```python
from build123d import *

# Parameters (mm, degrees)
ESQUISSE1_W             = 130.51
ESQUISSE1_H             = 72.96
BOSS_EXTRU_4_DEPTH      = 4
ESQUISSE5_W             = 128.51
ESQUISSE5_H             = 70.96
ENL_V_MAT_EXTRU_1_DEPTH = 1.36
ESQUISSE6_W             = 60.96
ESQUISSE6_H             = 1.36
ENL_V_MAT_EXTRU_2_DEPTH = 149.70104808
ESQUISSE12_W            = 5.045005
ESQUISSE12_H            = 5
BOSS_EXTRU_10_DEPTH     = 4
ESQUISSE14_W            = 2
ESQUISSE14_H            = 5
BOSS_EXTRU_11_DEPTH     = 8
ESQUISSE15_W            = 2
ESQUISSE15_H            = 6
BOSS_EXTRU_12_DEPTH     = 8
ESQUISSE16_W            = 2
ESQUISSE16_H            = 6
BOSS_EXTRU_13_DEPTH     = 8
ESQUISSE17_W            = 5.045005
ESQUISSE17_H            = 5
BOSS_EXTRU_14_DEPTH     = 4
ESQUISSE19_W            = 2
ESQUISSE19_H            = 5
BOSS_EXTRU_15_DEPTH     = 8


with BuildPart() as part:
    # Esquisse1 → Boss.-Extru.4 (new body)
    with BuildSketch(Plane(origin=(0, 0, 0), x_dir=(1, 0, 0), z_dir=(0, 1, 0))):
        with Locations((65.255, 36.48)):
            Rectangle(ESQUISSE1_W, ESQUISSE1_H)
    extrude(amount=BOSS_EXTRU_4_DEPTH)

    # Esquisse5 → Enlèv. mat.-Extru.1 (cut)
    with BuildSketch(Plane(origin=(0, 4, 0), x_dir=(1, 0, 0), z_dir=(0, 1, 0))):
        with Locations((65.255, 36.48)):
            Rectangle(ESQUISSE5_W, ESQUISSE5_H)
    extrude(amount=-ENL_V_MAT_EXTRU_1_DEPTH, mode=Mode.SUBTRACT)

    # Esquisse6 → Enlèv. mat.-Extru.2 (cut, through all)
    with BuildSketch(Plane.ZY.offset(-129.51)):
        with Locations((-36.48, 3.32)):
            Rectangle(ESQUISSE6_W, ESQUISSE6_H)
    extrude(amount=-ENL_V_MAT_EXTRU_2_DEPTH, mode=Mode.SUBTRACT)

    # Esquisse12 → Boss.-Extru.10 (add)
    with BuildSketch(Plane.XZ):
        with Locations((133.0325025, -70.46)):
            Rectangle(ESQUISSE12_W, ESQUISSE12_H)
        with Locations((133.0325025, -2.5)):
            Rectangle(ESQUISSE12_W, ESQUISSE12_H)
    extrude(amount=-BOSS_EXTRU_10_DEPTH)

    # Esquisse14 → Boss.-Extru.11 (add)
    with BuildSketch(Plane(origin=(0, 4, 0), x_dir=(1, 0, 0), z_dir=(0, 1, 0))):
        with Locations((134.555005, 70.46)):
            Rectangle(ESQUISSE14_W, ESQUISSE14_H)
        with Locations((134.555005, 2.5)):
            Rectangle(ESQUISSE14_W, ESQUISSE14_H)
    extrude(amount=BOSS_EXTRU_11_DEPTH)

    # Esquisse15 → Boss.-Extru.12 (add)
    with BuildSketch(Plane(origin=(0, 0, -5), x_dir=(-1, 0, 0), z_dir=(0, 0, -1))):
        with Locations((-134.555005, 9)):
            Rectangle(ESQUISSE15_W, ESQUISSE15_H)
    extrude(amount=BOSS_EXTRU_12_DEPTH)

    # Esquisse16 → Boss.-Extru.13 (add)
    with BuildSketch(Plane.XY.offset(-67.96)):
        with Locations((134.555005, 9)):
            Rectangle(ESQUISSE16_W, ESQUISSE16_H)
    extrude(amount=BOSS_EXTRU_13_DEPTH)

    # Esquisse17 → Boss.-Extru.14 (add)
    with BuildSketch(Plane.XZ):
        with Locations((-2.5225025, -52.46)):
            Rectangle(ESQUISSE17_W, ESQUISSE17_H)
        with Locations((-2.5225025, -20.5)):
            Rectangle(ESQUISSE17_W, ESQUISSE17_H)
    extrude(amount=-BOSS_EXTRU_14_DEPTH)

    # Esquisse19 → Boss.-Extru.15 (add)
    with BuildSketch(Plane(origin=(0, 4, 0), x_dir=(1, 0, 0), z_dir=(0, 1, 0))):
        with Locations((-4.045005, 52.46)):
            Rectangle(ESQUISSE19_W, ESQUISSE19_H)
        with Locations((-4.045005, 20.5)):
            Rectangle(ESQUISSE19_W, ESQUISSE19_H)
    extrude(amount=BOSS_EXTRU_15_DEPTH)


solid = part.part
```
The listing builds one solid part. Answer for the finished solid, in the listing's coordinates (mm). A direction names the side the tool comes from. Coordinates: 2 decimals unless noted, no trailing zeros. Write each loop counter-clockwise with the first axis right and the second up, starting at its lowest first coordinate (ties: lowest second). Pieces come first, ordered by that corner, then holes. Notation, with made-up numbers: M 41,58.25 L 74,58.25 A37 cw 74,96.25 Z; hole C 35,80.25 d8. An arc over 180 degrees is marked long. Use a Markdown table: item, result. Add a question column.
1. Section C-C (x = 73) is taken. Give the vertices of the cut face in (y, z), plus the area to 3 significant figures.
2. Given P1, Ø5.5, axis at x = -1.5, y = 6.5, coming from the -Z side; P2, Ø1.6, axis at x = 135, z = -65.5, coming from the -Y side; P3, Ø2, axis at y = 2.5, z = -32, coming from the -X side; P4, Ø1.5, axis at x = 16, z = -33.5, coming from the -Y side, each flat-ended and moving along its own axis, determine where each tip first touches the part or whether it passes through.
3. Section D-D (z = -48) is taken. Give the vertices of the cut face in (x, y), plus the area to 3 significant figures.
4. Straight lines are drawn through the part: line 1 along Z through (x, y) = (59.5, 3.75); line 2 along X through (y, z) = (3.25, -68) (3 decimals); line 3 along Y through (x, z) = (14, -6.5). For each, find the intervals that lie inside material, in ascending order. Write a range as [from, to].
5. Which of the six approach directions +Z, -Z, +X, -X, +Y, -Y give full straight-line access (tool end or side, diameter ignored) to faces 1 (the flat face through (-4, 5, -23)), 2 (the flat face through (130.51, 1, -36)), 3 (the flat face through (0, 2, -64)), 4 (the flat face through (-3.045, 8, -52))?
6. Section B-B (z = -63.5) is taken. Give the vertices of the cut face in (x, y) (3 decimals).
7. Section A-A (y = 9) is taken. Give the vertices of the cut face in (x, z) (3 decimals).
8. For a pull along Z with two mould halves and no side action, classify faces 5 (the flat face through (0, 2, -9)), 6 (the flat face through (-4, 5, -54.96)), 7 (the flat face through (133, 2, -5)) as +Z half, -Z half, draft (parallel to the pull), parting line (faces both ways), or undercut.
Data:
| question | item | result |
|---|---|---|
| 1 | outline | M 0,-72.96 L 4,-72.96 L 4,-71.96 L 2.64,-71.96 L 2.64,-1 L 4,-1 L 4,0 L 0,0 Z |
| 1 | area | 195 mm2 |
| 2 | P1 | stops at z = -54.96 |
| 2 | P2 | stops at y = 6 |
| 2 | P3 | stops at x = 0 |
| 2 | P4 | stops at y = 0 |
| 3 | outline | M 0,0 L 130.51,0 L 130.51,2.64 L 1,2.64 L 1,4 L 0,4 Z |
| 3 | area | 346 mm2 |
| 4 | line 1 | z = [-72.96, -71.96], [-1, 0] |
| 4 | line 2 | x = [0, 1], [129.51, 135.555] |
| 4 | line 3 | y = [0, 2.64] |
| 5 | face 1 | -X, +Y, -Y |
| 5 | face 2 | +X, +Y, -Y |
| 5 | face 3 | -Z, -X, +Y, -Y |
| 5 | face 4 | +Z, -Z, +X, +Y |
| 6 | outline | M 0,0 L 130.51,0 L 130.51,2.64 L 1,2.64 L 1,4 L 0,4 Z; M 133.555,6 L 135.555,6 L 135.555,12 L 133.555,12 Z |
| 7 | outline | M -5.045,-54.96 L -3.045,-54.96 L -3.045,-49.96 L -5.045,-49.96 Z; M -5.045,-23 L -3.045,-23 L -3.045,-18 L -5.045,-18 Z; M 133.555,-72.96 L 135.555,-72.96 L 135.555,-59.96 L 133.555,-59.96 Z; M 133.555,-13 L 135.555,-13 L 135.555,0 L 133.555,0 Z |
| 8 | face 5 | draft |
| 8 | face 6 | -Z half |
| 8 | face 7 | undercut |
